```python
from build123d import *

# Parameters (mm, degrees)
SKETCH_1_W          = 54
SKETCH_1_H          = 20
EXTRUDE_1_DEPTH     = 37
SKETCH_2_W          = 67.922695334
SKETCH_2_H          = 39.407561178
SKETCH_2_W_2        = 40
SKETCH_2_H_2        = 20
CUT_EXTRUDE_1_DEPTH = 28
SKETCH_3_W          = 67.922695334
SKETCH_3_H          = 33.385731604
SKETCH_3_W_2        = 40
SKETCH_3_H_2        = 20
CUT_EXTRUDE_2_DEPTH = 6
FILLET_1_R          = 1
FILLET_2_R          = 2
CHAMFER_1_SIZE      = 1
CHAMFER_1_SIZE2     = 2
SKETCH_4_R          = 2
CUT_EXTRUDE_3_DEPTH = 30
RIB_1_REACH         = 48.883
SKETCH_5_WALL_W     = 99.888770984
SKETCH_5_WALL_H     = 1
EXTRUDE_START       = -1
EXTRUDE_4_DEPTH     = 3
SKETCH_9_R          = 6.5
EXTRUDE_5_DEPTH     = 2
CUT_EXTRUDE_START   = -0.5
SKETCH_10_R         = 6.5
SKETCH_10_R_2       = 5
CUT_EXTRUDE_4_DEPTH = 0.5
SKETCH_11_R         = 3
EXTRUDE_6_DEPTH     = 4
SKETCH_14_R         = 1.5
CUT_EXTRUDE_5_DEPTH = 4
SCALE_1_SCALE       = 0.5


with BuildPart() as part:
    # 草图1 → 凸台-拉伸1 (new body)
    with BuildSketch(Plane(origin=(0, 0, 0), x_dir=(1, 0, 0), z_dir=(0, 1, 0))):
        Rectangle(SKETCH_1_W, SKETCH_1_H)
    extrude(amount=EXTRUDE_1_DEPTH)

    # 草图2 → 切除-拉伸1 (cut)
    with BuildSketch(Plane.XZ):
        Rectangle(SKETCH_2_W, SKETCH_2_H)
        Rectangle(SKETCH_2_W_2, SKETCH_2_H_2, mode=Mode.SUBTRACT)
    extrude(amount=-CUT_EXTRUDE_1_DEPTH, mode=Mode.SUBTRACT)

    # 草图3 → 切除-拉伸2 (cut)
    with BuildSketch(Plane(origin=(0, 37, 0), x_dir=(1, 0, 0), z_dir=(0, 1, 0))):
        Rectangle(SKETCH_3_W, SKETCH_3_H)
        Rectangle(SKETCH_3_W_2, SKETCH_3_H_2, mode=Mode.SUBTRACT)
    extrude(amount=-CUT_EXTRUDE_2_DEPTH, mode=Mode.SUBTRACT)

    # 圆角1
    fillet_1_edges = [part.edges().sort_by_distance(p)[0] for p in [
        (20, 14, -10),
        (-20, 14, -10),
        (-20, 14, 10),
        (20, 14, 10),
        (0, 37, -10),
        (0, 37, 10),
        (20, 37, 0),
        (20, 34, 10),
        (-20, 34, 10),
        (-20, 37, 0),
        (-20, 34, -10),
        (20, 34, -10),
    ]]
    fillet(fillet_1_edges, radius=FILLET_1_R)

    # 圆角2
    fillet_2_edges = [part.edges().sort_by_distance(p)[0] for p in [
        (27, 29.5, 10),
        (-27, 29.5, 10),
        (-27, 29.5, -10),
        (27, 29.5, -10),
    ]]
    fillet(fillet_2_edges, radius=FILLET_2_R)

    # 倒角1
    chamfer_1_edges = [part.edges().sort_by_distance(p)[0] for p in [
        (0, 0, -10),
        (0, 0, 10),
        (-20, 0, 0),
        (20, 0, 0),
        (-19.707106781, 0, 9.707106781),
        (19.707106781, 0, 9.707106781),
        (19.707106781, 0, -9.707106781),
        (-19.707106781, 0, -9.707106781),
    ]]
    chamfer_1_side = [part.faces().sort_by_distance(p)[0] for p in [
        (0, 0, 0),
    ]]
    chamfer(chamfer_1_edges, length=CHAMFER_1_SIZE, length2=CHAMFER_1_SIZE2, reference=chamfer_1_side[0])

    # 草图4 → 切除-拉伸3 (cut)
    with BuildSketch(Plane(origin=(0, 37, 0), x_dir=(1, 0, 0), z_dir=(0, 1, 0))):
        with Locations(Location((-24, 5, 0), (0, 0, 270))):
            Circle(SKETCH_4_R)
        with Locations(Location((-24, -5, 0), (0, 0, 270))):
            Circle(SKETCH_4_R)
        with Locations(Location((24, -5, 0), (0, 0, 270))):
            Circle(SKETCH_4_R)
        with Locations(Location((24, 5, 0), (0, 0, 270))):
            Circle(SKETCH_4_R)
    extrude(amount=-CUT_EXTRUDE_3_DEPTH, mode=Mode.SUBTRACT)

    # 草图5 wall → 筋1 (add, up to next)
    with BuildSketch(Plane(origin=(-22, 31.5, 0), x_dir=(-0.970142500145, -0.242535625036, 0), z_dir=(0.242535625036, -0.970142500145, 0)), mode=Mode.PRIVATE) as rib_1_sk1:
        Rectangle(SKETCH_5_WALL_W, SKETCH_5_WALL_H)
    rib_1_tool1 = extrude(rib_1_sk1.sketch, amount=RIB_1_REACH, mode=Mode.PRIVATE) - part.part
    rib_1 = rib_1_tool1.solids().sort_by_distance((-22, 31.5, 0))[0]
    add(rib_1)

    # 镜向1: 筋1 across plane
    add(rib_1.mirror(Plane(origin=(0, 0, 0), x_dir=(0, 0, 1), z_dir=(1, 0, 0))))

    # 草图8 → 凸台-拉伸4 (add)
    with BuildSketch(Plane(origin=(0, 37, 0), x_dir=(1, 0, 0), z_dir=(0, 1, 0)).offset(EXTRUDE_START)):
        with BuildLine():
            Line((-15, 9.5), (6.877501001, 9.5))
            ThreePointArc((6.877501001, 9.5), (20, 0), (6.877501001, -9.5))
            Line((6.877501001, -9.5), (-15, -9.5))
            Line((-15, -9.5), (-15, -3))
            ThreePointArc((-15, -3), (-16, 0), (-15, 3))
            Line((-15, 3), (-15, 9.5))
        make_face()
    extrude(amount=EXTRUDE_4_DEPTH)

    # 草图9 → 凸台-拉伸5 (add)
    with BuildSketch(Plane(origin=(0, 39, 0), x_dir=(1, 0, 0), z_dir=(0, 1, 0))):
        with Locations(Location((10, 0, 0), (0, 0, 270))):
            Circle(SKETCH_9_R)
    extrude(amount=EXTRUDE_5_DEPTH)

    # 草图10 → 切除-拉伸4 (cut)
    with BuildSketch(Plane(origin=(0, 41, 0), x_dir=(1, 0, 0), z_dir=(0, 1, 0)).offset(CUT_EXTRUDE_START)):
        with Locations(Location((10, 0, 0), (0, 0, 270))):
            Circle(SKETCH_10_R)
        with Locations(Location((10, 0, 0), (0, 0, 270))):
            Circle(SKETCH_10_R_2, mode=Mode.SUBTRACT)
    extrude(amount=CUT_EXTRUDE_4_DEPTH, mode=Mode.SUBTRACT)

    # 草图11 → 凸台-拉伸6 (add)
    with BuildSketch(Plane(origin=(0, 41, 0), x_dir=(1, 0, 0), z_dir=(0, 1, 0))):
        with Locations(Location((10, 0, 0), (0, 0, 270))):
            Circle(SKETCH_11_R)
    extrude(amount=EXTRUDE_6_DEPTH)

    # 草图14 → 切除-拉伸5 (cut)
    with BuildSketch(Plane(origin=(0, 45, 0), x_dir=(1, 0, 0), z_dir=(0, 1, 0))):
        with Locations(Location((10, 0, 0), (0, 0, 270))):
            Circle(SKETCH_14_R)
    extrude(amount=-CUT_EXTRUDE_5_DEPTH, mode=Mode.SUBTRACT)


with BuildPart() as part_1:
    # 缩放比例1: scaled about (0.166200011, 19.802127708, 0)
    add(part.part.scale(SCALE_1_SCALE).moved(Location((0.083100006, 9.901063854, 0))))


solid = part_1.part
```
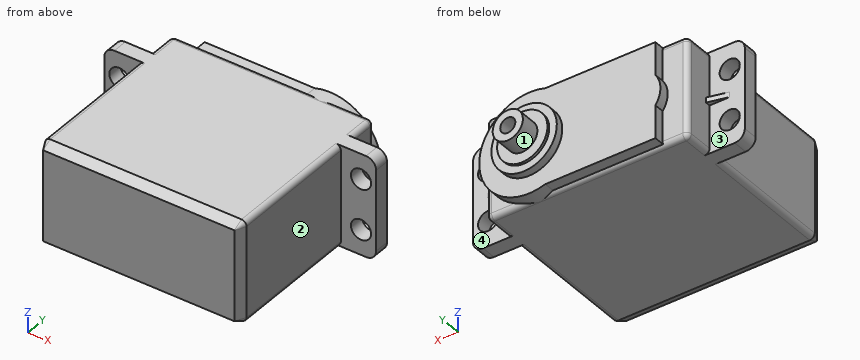
Work out the finished part from the listing and answer in its coordinate system (mm). Face numbers are marked on the shaded views. A direction names the side the tool comes from. Round coordinates to 2 decimals unless told otherwise and drop trailing zeros. Write each loop counter-clockwise with the first axis right and the second up, starting at its lowest first coordinate (ties: lowest second). Pieces come first, ordered by that corner, then holes. Notation, with made-up numbers: (4, 50.25) -> (60, 50.25) arc R22 ccw to (60, 57.25) -> close; hole circle Ø9 at (46.25, 5.5). An arc over 180 degrees is marked (long way). Write each question's results on one line, items separated by ' | '.
Q1. Flat-ended cylindrical pins translate along their axes: P1, Ø3, axis at x = -11, z = 0.5, coming from the +Y side; P2, Ø3, axis at y = 26.5, z = -1.5, coming from the -X side; P3, Ø3, axis at x = 12, z = 2, coming from the +Y side; P4, Ø1.5, axis at y = 19.5, z = -3.5, coming from the +X side. Find the tip coordinate at first contact, or state that the pin passes through.
Data:
P1: y = 28.39 | P2: x = -13.42 | P3: y = 25.4 | P4: x = 10.08
Q2. Which of the six approach directions +Z, -Z, +X, -X, +Y, -Y give full straight-line access (tool end or side, diameter ignored) to the marked faces 1, 2, 3 and 4?
Data:
face 1: +Y | face 2: +Z, -Z, +X, -Y | face 3: -X, +Y | face 4: +X, +Y
Q3. Section B-B, the plane x = -5.5 is taken. Write down the section's boundary in (y, z), then the cut area to 3 significant figures.
Data:
outline: (9.9, -4.5) -> (10.9, -5) -> (27.9, -5) arc R0.5 ccw to (28.33, -4.75) -> (29.4, -4.75) -> (29.4, 4.75) -> (28.33, 4.75) arc R0.5 ccw to (27.9, 5) -> (10.9, 5) -> (9.9, 4.5) -> close | area: 194 mm^2
Q4. Straight lines are drawn through the part: line 1 along X through (y, z) = (24.25, -2.5); line 2 along X through (y, z) = (31.7, 0); line 3 along Z through (x, y) = (11.5, 25.25). For each, find the intervals that lie inside material, in ascending order. Write a range as [from, to].
Data:
line 1: [-13.42, -12.92], [-10.92, 11.08], [13.08, 13.58] | line 2: [3.58, 4.33], [5.83, 6.58] | line 3: [-5, -3.31], [-1.69, 1.69], [3.31, 5]
Q5. Section A-A, the plane y = 11.75 is taken. Write down the section's boundary in (x, z).
Data:
outline: (-9.92, -4.5) arc R0.5 ccw to (-9.42, -5) -> (9.58, -5) arc R0.5 ccw to (10.08, -4.5) -> (10.08, 4.5) arc R0.5 ccw to (9.58, 5) -> (-9.42, 5) arc R0.5 ccw to (-9.92, 4.5) -> close
